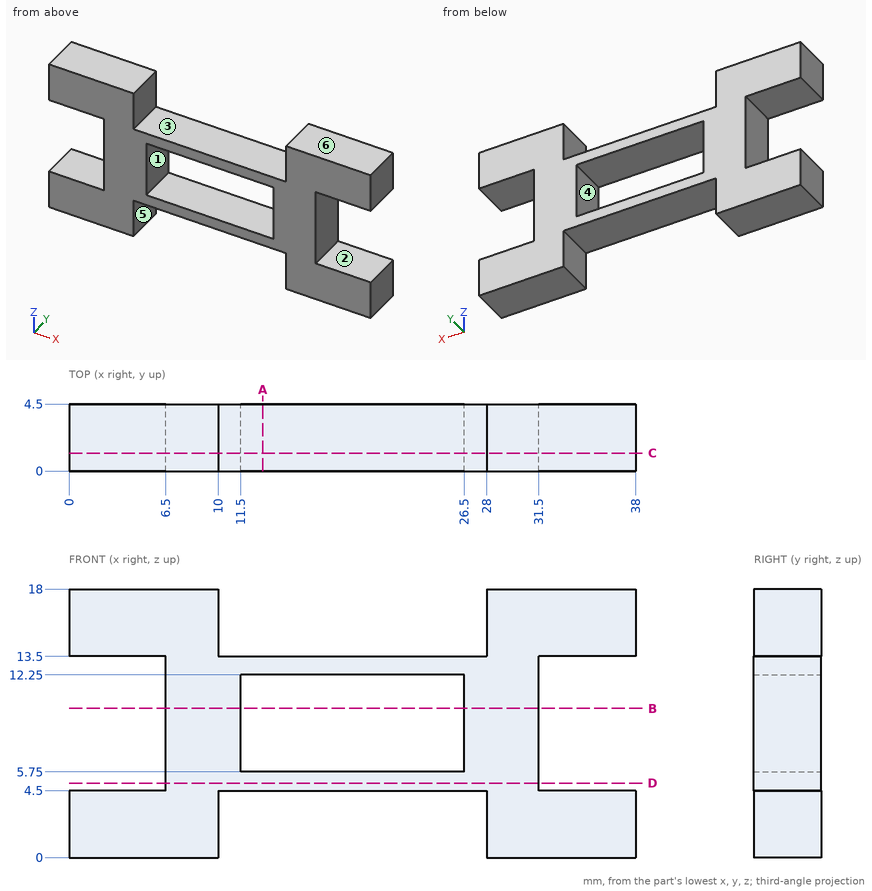
Geometry check sheet. Reference: drawing and pictorial views, mm from the part's lowest x, y, z. A direction names the side the tool comes from. Coordinates: 2 decimals unless noted, no trailing zeros. Loops run counter-clockwise (first coordinate to the right, second up) from the corner with the lowest first, then second, coordinate; pieces in that order, holes last. Notation, with made-up numbers: M -33.5,49 L -16.5,49 A31 cw -16.5,75 Z; hole C -25.75,24.5 d8. An arc over 180 degrees is marked long. One line per item, written item: value.
1. Gauge pin test, flat ends, axial feed: P1, Ø1.3, axis at y = 2.5, z = 2, coming from the -X side; P2, Ø2, axis at y = 1, z = 9, coming from the -X side; P3, Ø1.3, axis at y = 3, z = 10.5, coming from the +X side. Record the tip position at first contact, or that the pin passes through.
Answers follow:
P1: x = 0
P2: x = 6.5
P3: x = 31.5
2. Set-up check for the marked faces 1, 2 and 3: record each of +Z, -Z, +X, -X, +Y, -Y from which the full face is reachable in a straight line by a thin tool's end or side.
Answers follow:
face 1: +Y, -Y
face 2: +X, +Y, -Y
face 3: +Z, +Y, -Y
3. Section check D-D on z = 5. Record the cut outline in (x, y).
Answers follow:
outline: M 6.5,0 L 31.5,0 L 31.5,4.5 L 6.5,4.5 Z
4. Section check C-C on y = 1.2. Record the cut outline in (x, z), plus the area to 4 significant figures.
Answers follow:
outline: M 0,0 L 10,0 L 10,4.5 L 28,4.5 L 28,0 L 38,0 L 38,4.5 L 31.5,4.5 L 31.5,13.5 L 38,13.5 L 38,18 L 28,18 L 28,13.5 L 10,13.5 L 10,18 L 0,18 L 0,13.5 L 6.5,13.5 L 6.5,4.5 L 0,4.5 Z; hole M 11.5,5.75 L 26.5,5.75 L 26.5,12.25 L 11.5,12.25 Z
area: 307.5 mm^2
5. Mould release check, pull along Z, two halves, no side actions. Record for the marked faces 4, 5 and 6: pulls with the +Z half, pulls with the -Z half, needs draft (parallel to the pull), parting line crosses it, or undercut.
Answers follow:
face 4: undercut
face 5: needs draft
face 6: pulls with the +Z half
6. Section check B-B on z = 10. Record the cut outline in (x, y).
Answers follow:
outline: M 6.5,0 L 11.5,0 L 11.5,4.5 L 6.5,4.5 Z; M 26.5,0 L 31.5,0 L 31.5,4.5 L 26.5,4.5 Z
7. Section check A-A on x = 13. Record the cut outline in (y, z).
Answers follow:
outline: M 0,4.5 L 4.5,4.5 L 4.5,5.75 L 0,5.75 Z; M 0,12.25 L 4.5,12.25 L 4.5,13.5 L 0,13.5 Z
8. Material ranges on line 1 along X through (y, z) = (1.5, 1.75); line 2 along X through (y, z) = (1.25, 8.5); line 3 along Z through (x, y) = (26, 3.1), recorded low to high. Write a range as from..to.
Answers follow:
line 1: 0..10, 28..38
line 2: 6.5..11.5, 26.5..31.5
line 3: 4.5..5.75, 12.25..13.5
